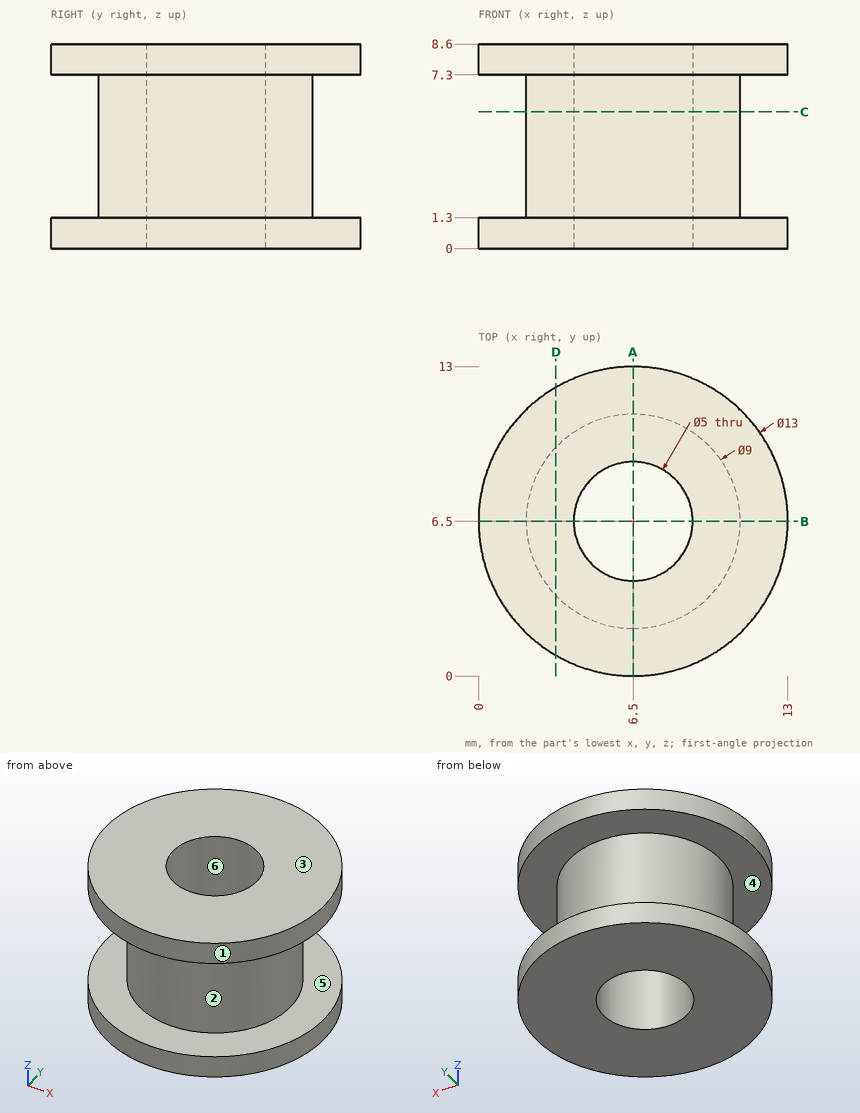
The figure shows three views and two pictorial views of one solid part (mm, origin at its lowest corner). Answer the questions. A direction names the side the tool comes from. Round coordinates to 2 decimals unless told otherwise and drop trailing zeros. Write each loop counter-clockwise with the first axis right and the second up, starting at its lowest first coordinate (ties: lowest second). Pieces come first, ordered by that corner, then holes. Notation, with made-up numbers: (-17.75, 54) - (-4.75, 54) arc R10 ccw to (-4.75, 68) - close; hole circle Ø7 at (76, 7). An arc over 180 degrees is marked (long way). Answer in a Markdown table with one row per item. Add a question column.
1. Find the intervals of material crossed by line 1 along X through (y, z) = (6.5, 6.5); line 2 along Z through (x, y) = (11, 4.5); line 3 along X through (y, z) = (8, 1), in increasing order. Write a range as from..to.
2. A cutting plane is placed at A-A, the plane x = 6.5. Determine the outline of the cut face in (y, z), and give its area (3 significant figures).
3. The mould has two halves that part along Z. Classify the marked faces 3, 4, 5 and 6: +Z half, -Z half, draft (parallel to the pull), parting line (faces both ways), or undercut.
4. A cutting plane is placed at D-D, the plane x = 3.25. Determine the outline of the cut face in (y, z).
5. For the marked faces 1 and 2, determine the directions among +Z, -Z, +X, -X, +Y, -Y from which every point of the face is accessible in a straight line to the end or side of a thin tool.
6. Given pin 1 (3 mm diameter, centred on x = 6.5, y = 6.5, fed in from -Z); pin 2 (4 mm diameter, centred on y = 2.5, z = 7, fed in from +X); pin 3 (5 mm diameter, centred on y = 1.5, z = 6, fed in from +X); pin 4 (1 mm diameter, centred on y = 9.5, z = 3, fed in from -X), each flat-ended and moving along its own axis, determine where each tip first touches the part or whether it passes through.
7. A cutting plane is placed at C-C, the plane z = 5.75. Determine the outline of the cut face in (x, y), and give its area (3 significant figures).
Worked out:
| question | item | result |
|---|---|---|
| 1 | line 1 | 2..4, 9..11 |
| 1 | line 2 | 0..1.3, 7.3..8.6 |
| 1 | line 3 | 0.18..4.5, 8.5..12.82 |
| 2 | outline | (0, 0) - (4, 0) - (4, 8.6) - (0, 8.6) - (0, 7.3) - (2, 7.3) - (2, 1.3) - (0, 1.3) - close; (9, 0) - (13, 0) - (13, 1.3) - (11, 1.3) - (11, 7.3) - (13, 7.3) - (13, 8.6) - (9, 8.6) - close |
| 2 | area | 44.8 mm^2 |
| 3 | face 3 | +Z half |
| 3 | face 4 | undercut |
| 3 | face 5 | undercut |
| 3 | face 6 | draft |
| 4 | outline | (0.87, 0) - (12.13, 0) - (12.13, 1.3) - (9.61, 1.3) - (9.61, 7.3) - (12.13, 7.3) - (12.13, 8.6) - (0.87, 8.6) - (0.87, 7.3) - (3.39, 7.3) - (3.39, 1.3) - (0.87, 1.3) - close |
| 5 | face 1 | +Z, -Z |
| 5 | face 2 | none |
| 6 | pin 1 | through |
| 6 | pin 2 | x = 12.68 |
| 6 | pin 3 | x = 12.33 |
| 6 | pin 4 | x = 2.76 |
| 7 | outline | circle Ø9 at (6.5, 6.5); hole circle Ø5 at (6.5, 6.5) |
| 7 | area | 44.0 mm^2 |
